Geometry: final body of the model. Coordinates: model frame, mm. Face numbers are marked on the shaded views. A direction names the side the tool comes from. Give positions to 0.01 mm unless a question says otherwise; leave off trailing zeros. Loops run counter-clockwise (first coordinate to the right, second up) from the corner with the lowest first, then second, coordinate; pieces in that order, holes last. Notation, with made-up numbers: (11.25, 47) -> (21.25, 47) arc R13 ccw to (21.25, 70) -> close; hole circle Ø7 at (64.5, 82). An arc over 180 degrees is marked (long way). Answer in a Markdown table with one row per item. Add a question column.
1) Draft query along X for the marked faces 4, 5, 6 and 7. Return one class per face: +X half, -X half, draft (parallel to the pull), parting line (faces both ways), or undercut.
2) Section query B-B (y = 18). Return the cut outline in (x, z).
3) Line query: line 1 (Z direction, x = 0, y = 29); line 2 (Z direction, x = 14, y = 8.5); line 3 (Z direction, x = -5.5, y = 25). Output: solid intervals per line, ascending. Write a range as from..to.
4) Section query D-D (z = 40). Return the cut outline in (x, y).
5) First-contact query: P1, Ø1, axis at x = 42, z = 17, coming from the -Y side; P2, Ø6, axis at x = 19, z = 28, coming from the -Y side; P3, Ø2, axis at x = -6.5, y = 24.5, coming from the +Z side. Flat tips, straight axial feed; report the tip coordinate or a pass-through.
6) Access query for the marked faces 1, 2 and 3. Directions: +Z, -Z, +X, -X, +Y, -Y. A direction counts if a zero-diameter tool reaches every point of the face in a straight line with its end or side. Return the directions, or none.
7) Section query A-A (x = -6). Return the cut outline in (y, z).
8) Section query C-C (x = 48.5). Return the cut outline in (y, z).
```python
from build123d import *

# Parameters (mm, degrees)
F0_W     = 83.440322
F0_H     = 90.671822
F1_DEPTH = 50.8
F3_DEPTH = 83.441322
F4_R     = 8.441075
F5_DEPTH = 90.672822
F7_DEPTH = 12.7
F8_SIZE  = 50.8


with BuildPart() as f1:
    # F0 (on Top) → F1 (new body)
    with BuildSketch(Plane.XY):
        with Locations((1.29796, 0)):
            Rectangle(F0_W, F0_H)
    extrude(amount=F1_DEPTH)

    # F2 (on face) → F3 (cut, through all)
    with BuildSketch(Plane(origin=(-40.422201, 0, 0), x_dir=(0, -1, 0), z_dir=(-1, 0, 0))):
        Polygon((45.335911, 50.8), (0, 50.8), (45.335911, 0), align=None)
    extrude(amount=-F3_DEPTH, mode=Mode.SUBTRACT)

    # F4 (on face) → F5 (cut, through all)
    with BuildSketch(Plane(origin=(0, 45.335911, 0), x_dir=(-1, 0, 0), z_dir=(0, 1, 0))):
        with Locations((0, 26.879085)):
            Circle(F4_R)
    extrude(amount=-F5_DEPTH, mode=Mode.SUBTRACT)

    # F6 (on face) → F7 (join)
    with BuildSketch(Plane.YZ.offset(43.018121)):
        Polygon((-45.335911, 0), (45.335911, 0), (45.335911, 50.8), (0, 50.8), align=None)
        Polygon((-52.660115, 0), (-45.335911, 0), (0, 50.8), (45.335911, 50.8), (45.335911, 60.355168), (-52.660115, 60.355168), align=None)
    extrude(amount=F7_DEPTH)

    # F8
    f8_edges = [f1.edges().sort_by_distance(p)[0] for p in [
        (49.368121, -52.660115, 60.355168),
    ]]
    chamfer(f8_edges, length=F8_SIZE)


solid = f1.part
```
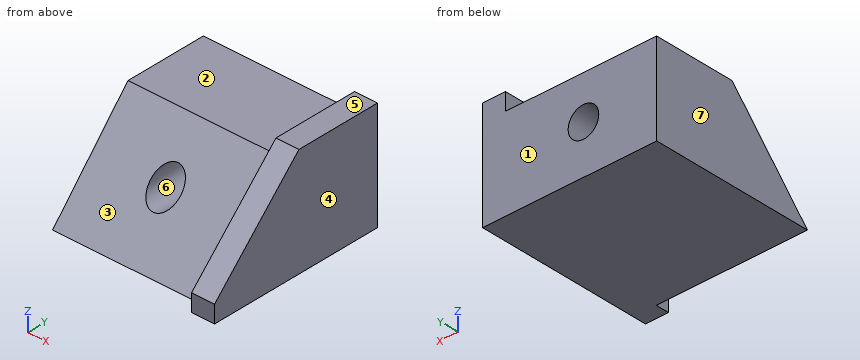
Evaluation:
| question | item | result |
|---|---|---|
| 1 | face 4 | +X half |
| 1 | face 5 | draft |
| 1 | face 6 | undercut |
| 1 | face 7 | -X half |
| 2 | outline | (-40.42, 0) -> (55.72, 0) -> (55.72, 60.36) -> (43.02, 60.36) -> (43.02, 50.8) -> (-40.42, 50.8) -> close; hole circle Ø16.88 at (0, 26.88) |
| 3 | line 1 | 0..18.44, 35.32..50.8 |
| 3 | line 2 | 0..50.8 |
| 3 | line 3 | 0..20.48, 33.28..50.8 |
| 4 | outline | (-40.42, -9.64) -> (43.02, -9.64) -> (43.02, -22.22) -> (55.72, -22.22) -> (55.72, 45.34) -> (-40.42, 45.34) -> close |
| 5 | P1 | y = -30.61 |
| 5 | P2 | y = -23.02 |
| 5 | P3 | z = 50.8 |
| 6 | face 1 | +Z, -Z, +X, -X, +Y |
| 6 | face 2 | +Z, -X, +Y, -Y |
| 6 | face 3 | +Z, -X, -Y |
| 7 | outline | (-45.34, 0) -> (45.34, 0) -> (45.34, 20.94) -> (-26.65, 20.94) -> close; (-16.05, 32.82) -> (45.34, 32.82) -> (45.34, 50.8) -> (0, 50.8) -> close |
| 8 | outline | (-52.66, 0) -> (45.34, 0) -> (45.34, 60.36) -> (-1.86, 60.36) -> (-52.66, 9.56) -> close |
